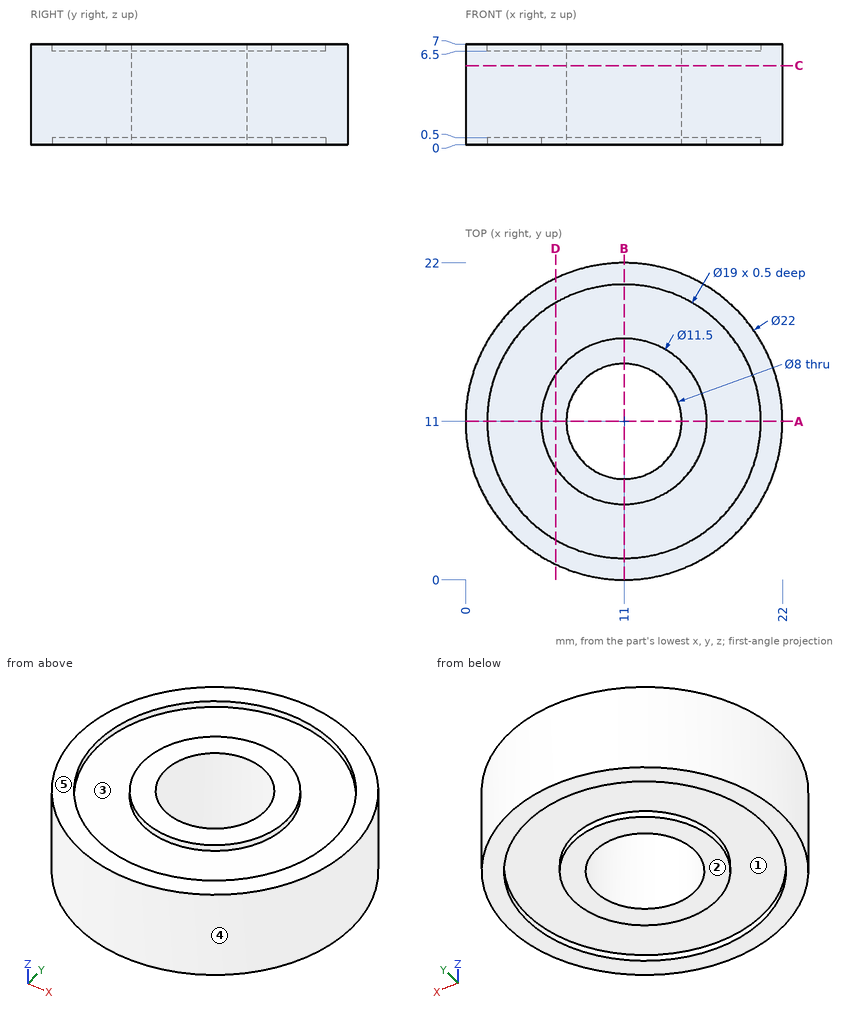
Job drawing, mm, ordinate dimensions from the low corner. One solid piece. A direction names the side the tool comes from. Round coordinates to 2 decimals unless told otherwise and drop trailing zeros. Write each loop counter-clockwise with the first axis right and the second up, starting at its lowest first coordinate (ties: lowest second). Pieces come first, ordered by that corner, then holes. Notation, with made-up numbers: M 13.25,87.25 L 69.25,87.25 A28 ccw 69.25,111.25 Z; hole C 64.5,33 d2. An arc over 180 degrees is marked long. Return JSON: item names as keys, results as strings. Group by question number.
(1) Two-plate mould, pull along Y, no slides. Class the marked faces 3, 4 and 5: +Y half, -Y half, draft (parallel to the pull), parting line (faces both ways), or undercut.
(2) Saw through at D-D on x = 6.25. Write the cut outline in (y, z).
(3) Saw through at A-A on y = 11. Write the cut outline in (x, z).
(4) Which spindle directions (+Z, -Z, +X, -X, +Y, -Y) get a long thin tool onto all of the face, cutting with end or side? Do the marked faces 1 and 2. Say none if no direction does.
(5) Drill centre lines: probe 1 along Y at (x, z) = (11, 6.95); probe 2 along Z at (x, y) = (7.75, 18.75); probe 3 along Y at (x, z) = (12, 2.5). Where is each one in solid material? Low to high.
(6) Pin check, flat tips, straight feed: pin 1 Ø2 at (x, y) = (4.5, 6) entering from -Z; pin 2 Ø10.5 at (x, y) = (11, 11) entering from -Z; pin 3 Ø1 at (x, z) = (19.5, 4) entering from -Y; pin 4 Ø4 at (y, z) = (7.5, 5) entering from +X. Stop position of each tip, or through.
(7) Saw through at C-C on z = 5.5. Write the cut outline in (x, y).
Returned:
{
 "1": {"face 3": "undercut", "face 4": "parting line", "face 5": "draft"},
 "2": {"outline": "M 1.08,0 L 2.77,0 L 2.77,0.5 L 7.76,0.5 L 7.76,0 L 14.24,0 L 14.24,0.5 L 19.23,0.5 L 19.23,0 L 20.92,0 L 20.92,7 L 19.23,7 L 19.23,6.5 L 14.24,6.5 L 14.24,7 L 7.76,7 L 7.76,6.5 L 2.77,6.5 L 2.77,7 L 1.08,7 Z"},
 "3": {"outline": "M 0,0 L 1.5,0 L 1.5,0.5 L 5.25,0.5 L 5.25,0 L 7,0 L 7,7 L 5.25,7 L 5.25,6.5 L 1.5,6.5 L 1.5,7 L 0,7 Z; M 15,0 L 16.75,0 L 16.75,0.5 L 20.5,0.5 L 20.5,0 L 22,0 L 22,7 L 20.5,7 L 20.5,6.5 L 16.75,6.5 L 16.75,7 L 15,7 Z"},
 "4": {"face 1": "-Z", "face 2": "-Z, +X, -X, +Y, -Y"},
 "5": {"probe 1": "0 to 1.5, 5.25 to 7, 15 to 16.75, 20.5 to 22", "probe 2": "0.5 to 6.5", "probe 3": "0.05 to 7.13, 14.87 to 21.95"},
 "6": {"pin 1": "z = 0.5", "pin 2": "z = 0", "pin 3": "y = 3.45", "pin 4": "x = 21.9"},
 "7": {"outline": "C 11,11 d22; hole C 11,11 d8"}
}
